Design review of the part built by this model. Coordinates are the model's own, in mm. Face numbers are marked on the shaded views. Give positions to 0.01 mm unless a question says otherwise; leave off trailing zeros. Write each loop counter-clockwise with the first axis right and the second up, starting at its lowest first coordinate (ties: lowest second). Pieces come first, ordered by that corner, then holes.
```python
from build123d import *

# Parameters (mm, degrees)
SKETCH1_W               = 23.8125
SKETCH1_H               = 15.875
BASE_FLANGE1_DEPTH      = 6.35
F_1_4_20_TAPPED_HOLE1_D = 5.1054
BREAK_CORNER1_DEPTH     = 6.35


# Read off the part's stored shape, not the designer's step: Break-Corner1
# Sheet-metal steps are written as plain solids
with BuildPart() as part:
    # Sketch1 → Base-Flange1 (new body)
    with BuildSketch(Plane.XY):
        Rectangle(SKETCH1_W, SKETCH1_H)
    extrude(amount=BASE_FLANGE1_DEPTH)

    # 1/4-20 Tapped Hole1 (through all)
    with Locations(Plane.XY.offset(6.35)):
        with Locations((0, 0)):
            Hole(F_1_4_20_TAPPED_HOLE1_D / 2)

    # Break-Corner1 outline → Break-Corner1 (cut)
    with BuildSketch(Plane.XY):
        with BuildLine():
            Line((-11.90625, -7.9375), (-8.73125, -7.9375))
            ThreePointArc((-8.73125, -7.9375), (-10.97631403, -7.00756403), (-11.90625, -4.7625))
            Line((-11.90625, -4.7625), (-11.90625, -7.9375))
        make_face()
        with BuildLine():
            ThreePointArc((11.90625, -4.7625), (10.97631403, -7.00756403), (8.73125, -7.9375))
            Line((8.73125, -7.9375), (11.90625, -7.9375))
            Line((11.90625, -7.9375), (11.90625, -4.7625))
        make_face()
        with BuildLine():
            Line((-11.90625, 7.9375), (-11.90625, 4.7625))
            ThreePointArc((-11.90625, 4.7625), (-10.97631403, 7.00756403), (-8.73125, 7.9375))
            Line((-8.73125, 7.9375), (-11.90625, 7.9375))
        make_face()
        with BuildLine():
            ThreePointArc((8.73125, 7.9375), (10.97631403, 7.00756403), (11.90625, 4.7625))
            Line((11.90625, 4.7625), (11.90625, 7.9375))
            Line((11.90625, 7.9375), (8.73125, 7.9375))
        make_face()
    extrude(amount=BREAK_CORNER1_DEPTH, mode=Mode.SUBTRACT)


solid = part.part
```
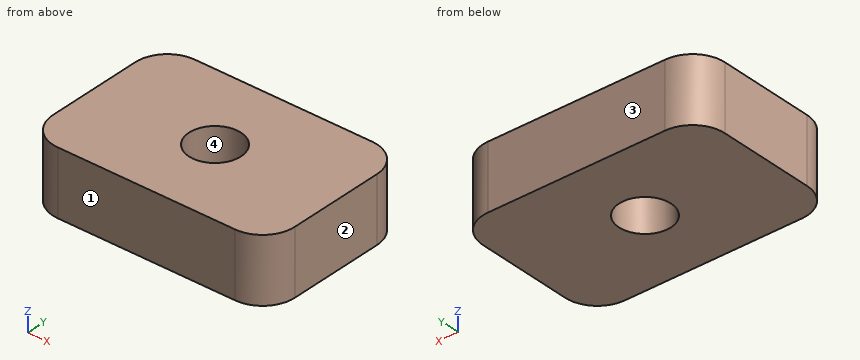
(1) Consider section A-A, the plane y = 0. Give the boundary of the cut face in (x, z), then the cut area to 3 significant figures.
Resolved:
outline: (-11.91, 0) - (-2.55, 0) - (-2.55, 6.35) - (-11.91, 6.35) - close; (2.55, 0) - (11.91, 0) - (11.91, 6.35) - (2.55, 6.35) - close
area: 119 mm2
(2) Consider section B-B, the plane x = 0. Give the boundary of the cut face in (y, z).
Resolved:
outline: (-7.94, 0) - (-2.55, 0) - (-2.55, 6.35) - (-7.94, 6.35) - close; (2.55, 0) - (7.94, 0) - (7.94, 6.35) - (2.55, 6.35) - close
(3) To check wall thickness, follow L1, parallel to Y at x = 0, z = 3.5; L2, parallel to Y at x = 0.5, z = 1.75; L3, parallel to X at y = -0.5, z = 1.75. State the ranges of each line that lie inside material, in increasing order.
Resolved:
L1: y = -7.94 to -2.55, 2.55 to 7.94
L2: y = -7.94 to -2.5, 2.5 to 7.94
L3: x = -11.91 to -2.5, 2.5 to 11.91
(4) Mouldability with a two-part tool opening along Y and no side actions: class the marked faces 1, 2, 3 and 4 as pulls with the +Y half, pulls with the -Y half, needs draft (parallel to the pull), parting line crosses it, or undercut.
Resolved:
face 1: pulls with the -Y half
face 2: needs draft
face 3: pulls with the +Y half
face 4: undercut
(5) Consider section D-D, the plane y = -6.5. Give the boundary of the cut face in (x, z), then the cut area to 3 significant figures.
Resolved:
outline: (-11.39, 0) - (11.39, 0) - (11.39, 6.35) - (-11.39, 6.35) - close
area: 145 mm2
